from build123d import *

# Parameters (mm, degrees)
SKETCH_2_W          = 6
SKETCH_2_H          = 15
CUT_EXTRUDE_1_DEPTH = 24


with BuildPart() as part:
    # 草图1 → 旋转1 (revolve)
    with BuildSketch(Plane.XY, mode=Mode.PRIVATE) as revolve_1_sk:
        with BuildLine():
            Line((-10, 28), (-10, 14.966629547))
            ThreePointArc((-10, 14.966629547), (-17.22497216, -5.22497216), (0, -18))
            Line((0, -18), (0, 28))
            Line((0, 28), (-10, 28))
        make_face()
    revolve(revolve_1_sk.sketch.rotate(Axis((0, 81.279546427, 0), (0, -1, 0)), 270), axis=Axis((0, 81.279546427, 0), (0, -1, 0)))

    # 草图2 → 切除-拉伸1 (cut)
    with BuildSketch(Plane(origin=(0, 28, 0), x_dir=(1, 0, 0), z_dir=(0, 1, 0))):
        Rectangle(SKETCH_2_W, SKETCH_2_H)
    extrude(amount=-CUT_EXTRUDE_1_DEPTH, mode=Mode.SUBTRACT)


solid = part.part
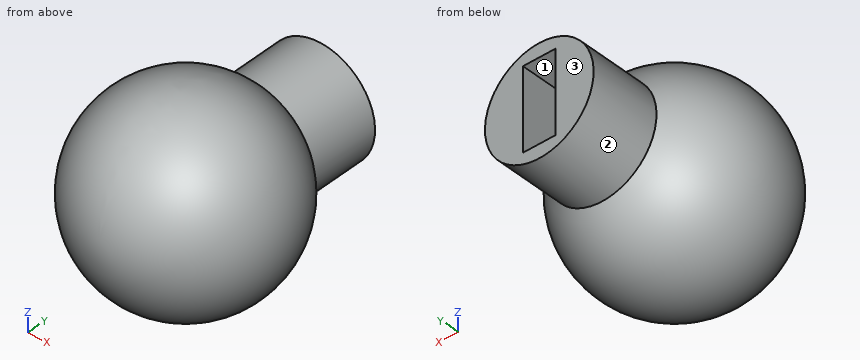
Part model, mm, in its own coordinate system. Face numbers are marked on the shaded views. Coordinates: 2 decimals unless noted, no trailing zeros. Loops run counter-clockwise (first coordinate to the right, second up) from the corner with the lowest first, then second, coordinate; pieces in that order, holes last. Notation, with made-up numbers: (29, 66) - (51, 66) arc R26 cw to (51, 95) - close; hole circle Ø3 at (39.5, 61). An arc over 180 degrees is marked (long way). Write each question's results on one line, items separated by ' | '. Start each with the question number.
Q1. Slice it at C-C on z = 2. Give the cut face in (x, y), and give its area (3 significant figures).
Q2. Probe line 1 along Z through (x, y) = (0.5, 20); line 2 along X through (y, z) = (5, -2); line 3 along X through (y, z) = (-8, 12). List the from-to ranges inside material, lowest first.
Q3. Slice it at A-A on y = 10. Give the cut face in (x, z).
Q4. Slice it at D-D on y = 24.5. Give the cut face in (x, z), and give its area (3 significant figures).
Q5. Drop flat-ended pins along their axis: pin 1 Ø5 at (x, z) = (-9.5, 5) entering from +Y; pin 2 Ø6 at (x, y) = (-2.5, 20.5) entering from -Z; pin 3 Ø5 at (x, z) = (14, -0.5) entering from +Y; pin 4 Ø6.5 at (x, y) = (-0.5, 12.5) entering from +Z. Give the stop position or say it passes through.
Q6. Two-plate mould, pull along X, no slides. Class the marked faces 1, 2 and 3: +X half, -X half, draft (parallel to the pull), parting line (faces both ways), or undercut.
Q7. Slice it at B-B on x = 0. Give the cut face in (y, z), and give its area (3 significant figures).
Answer:
1) outline: (-9.8, 14.97) arc R17.89 ccw (long way) to (9.8, 14.97) - (9.8, 28) - (3, 28) - (3, 4) - (-3, 4) - (-3, 28) - (-9.8, 28) - close | area: 1,080 mm2
2) line 1: z = -9.99 to -7.5, 7.5 to 9.99 | line 2: x = -17.18 to -3, 3 to 17.18 | line 3: x = -10.77 to 10.77
3) outline: circle Ø29.93 at (0, 0); hole (-3, -7.5) - (3, -7.5) - (3, 7.5) - (-3, 7.5) - close
4) outline: circle Ø20 at (0, 0); hole (-3, -7.5) - (3, -7.5) - (3, 7.5) - (-3, 7.5) - close | area: 224 mm2
5) pin 1: stops at y = 28 | pin 2: stops at z = -10 | pin 3: stops at y = 13.84 | pin 4: stops at z = 15.44
6) face 1: undercut | face 2: parting line | face 3: draft
7) outline: (4, -7.5) - (4, 7.5) - (28, 7.5) - (28, 10) - (14.97, 10) arc R18 ccw (long way) to (14.97, -10) - (28, -10) - (28, -7.5) - close | area: 877 mm2
